Verification items for this drawing (mm, ordinates from the low corner). A direction names the side the tool comes from. Round coordinates to 2 decimals unless told otherwise and drop trailing zeros. Write each loop counter-clockwise with the first axis right and the second up, starting at its lowest first coordinate (ties: lowest second). Pieces come first, ordered by that corner, then holes. Notation, with made-up numbers: (-39.5, -7.5) -> (8.5, -7.5) arc R6 ccw to (8.5, -0.5) -> close; hole circle Ø3 at (-24, 43). An arc over 180 degrees is marked (long way). One line per question, with ' | ' between items.
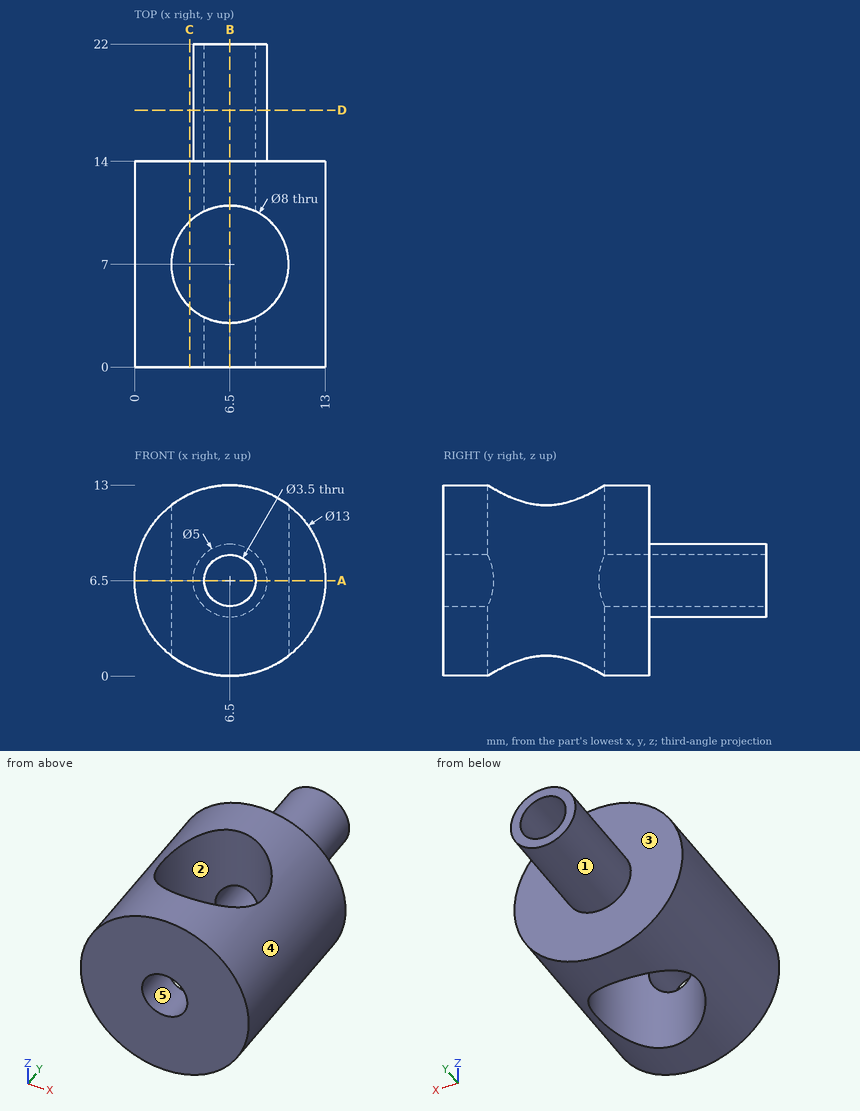
(1) Sectioned sample at C-C on x = 3.75. Record the cut outline in (y, z).
Resolved:
outline: (0, 0.61) -> (4.1, 0.61) -> (4.1, 12.39) -> (0, 12.39) -> close; (9.9, 0.61) -> (14, 0.61) -> (14, 12.39) -> (9.9, 12.39) -> close
(2) Draft check along X on the marked faces 3, 4 and 5. Enter one of: +X half, -X half, draft (parallel to the pull), parting line (faces both ways), or undercut.
Resolved:
face 3: draft | face 4: parting line | face 5: undercut
(3) Material ranges on line 1 (X direction, y = 17.5, z = 6.5); line 2 (X direction, y = 1.55, z = 6.5); line 3 (Y direction, x = 1, z = 7.25), recorded low to high.
Resolved:
line 1: x = 4 to 4.75, 8.25 to 9 | line 2: x = 0 to 4.75, 8.25 to 13 | line 3: y = 0 to 14
(4) Sectioned sample at D-D on y = 17.5. Record the cut outline in (x, z).
Resolved:
outline: circle Ø5 at (6.5, 6.5); hole circle Ø3.5 at (6.5, 6.5)
(5) Sectioned sample at A-A on z = 6.5. Record the cut outline in (x, y).
Resolved:
outline: (0, 0) -> (4.75, 0) -> (4.75, 3.4) arc R4 cw to (4.75, 10.6) -> (4.75, 22) -> (4, 22) -> (4, 14) -> (0, 14) -> close; (8.25, 0) -> (13, 0) -> (13, 14) -> (9, 14) -> (9, 22) -> (8.25, 22) -> (8.25, 10.6) arc R4 cw to (8.25, 3.4) -> close
(6) Go/stop test with flat-tipped pins: pin 1 (1.5 mm diameter, centred on y = 11, z = 8, fed in from +X); pin 2 (5 mm diameter, centred on y = 4, z = 1.5, fed in from -X); pin 3 (1 mm diameter, centred on x = 8.5, y = 17.5, fed in from -Z). Record where each tip stops, or that it passes through.
Resolved:
pin 1: stops at x = 12.96 | pin 2: stops at x = 0.5 | pin 3: stops at z = 4.5
(7) Sectioned sample at B-B on x = 6.5. Record the cut outline in (y, z), then the cut area to 3 significant figures.
Resolved:
outline: (0, 0) -> (3, 0) -> (3, 4.75) -> (0, 4.75) -> close; (0, 8.25) -> (3, 8.25) -> (3, 13) -> (0, 13) -> close; (11, 0) -> (14, 0) -> (14, 4) -> (22, 4) -> (22, 4.75) -> (11, 4.75) -> close; (11, 8.25) -> (22, 8.25) -> (22, 9) -> (14, 9) -> (14, 13) -> (11, 13) -> close | area: 69.0 mm2
(8) Access from +Z, -Z, +X, -X, +Y, -Y to the whole of each face (thin tool, end or side, straight path). Record for the marked faces 1 and 2.
Resolved:
face 1: +Y | face 2: +Z, -Z
